Geometry check sheet. Reference: the model listing, model coordinates, mm. Face numbers are marked on the shaded views. A direction names the side the tool comes from. Give positions to 0.01 mm unless a question says otherwise; leave off trailing zeros. Order: outer loops, then holes, each group sorted by start corner. A loop starts at its lowest first (then second) coordinate and runs counter-clockwise, first axis right, second up. Notation, with made-up numbers: M 13.25,-3 L 64.25,-3 A28 ccw 64.25,31 Z; hole C -2.5,79 d11. An arc over 180 degrees is marked long. Answer as a JSON object with one key per item and string values. Group by question number.
from build123d import *

# Parameters (mm, degrees)
CROQUIS1_W                   = 90
CROQUIS1_H                   = 50.8
SALIENTE_EXTRUIR1_DEPTH      = 6.35
TALADRO_DE_MARGEN_PARA_M61_D = 6.6
CROQUIS4_W                   = 38.1
CROQUIS4_H                   = 12.7
SALIENTE_EXTRUIR2_DEPTH      = 134.38


with BuildPart() as part:
    # Croquis1 → Saliente-Extruir1 (new, symmetric)
    with BuildSketch(Plane(origin=(0, 0, 0), x_dir=(1, 0, 0), z_dir=(0, 1, 0))):
        Rectangle(CROQUIS1_W, CROQUIS1_H)
    extrude(amount=SALIENTE_EXTRUIR1_DEPTH, both=True)

    # Taladro de margen para M61 (through all)
    with Locations(Plane(origin=(0, -6.35, 0), x_dir=(-1, 0, 0), z_dir=(0, -1, 0))):
        with Locations((-36.583684882, -75.725395139), (-37, -17), (-37, 17), (-3, -17), (-3, 17)):
            Hole(TALADRO_DE_MARGEN_PARA_M61_D / 2)

    # Croquis4 → Saliente-Extruir2 (add)
    with BuildSketch(Plane(origin=(0, 6.35, 0), x_dir=(1, 0, 0), z_dir=(0, 1, 0))):
        with Locations((-25.95, 19.05)):
            Rectangle(CROQUIS4_W, CROQUIS4_H)
    extrude(amount=SALIENTE_EXTRUIR2_DEPTH)


solid = part.part
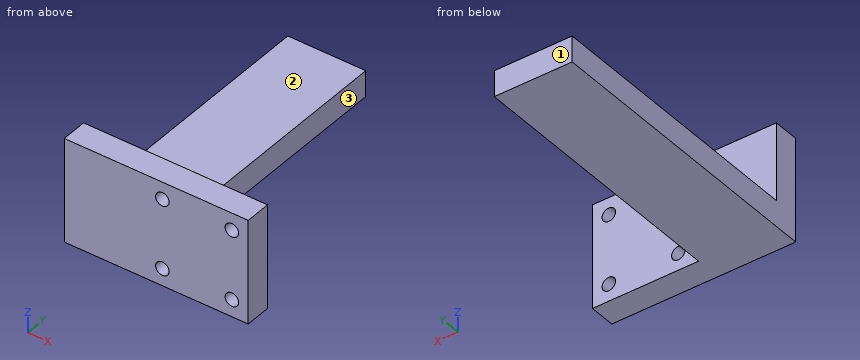
1. Thickness scan on line 1 along X through (y, z) = (2.5, 17); line 2 along Z through (x, y) = (37, 0); line 3 along X through (y, z) = (134, -17). Record the ranges inside material, lowest first. Write a range as [from, to].
2. Cross-section at A-A (z = -17). Record the cut outline in (x, y), and give its area (3 significant figures).
3. Access from +Z, -Z, +X, -X, +Y, -Y to the whole of each face (thin tool, end or side, straight path). Record for the marked faces 1, 2 and 3.
4. Cross-section at C-C (x = -18). Record the cut outline in (y, z), and give its area (3 significant figures).
5. Depth check by flat-ended pin: pin 1 (4 mm diameter, centred on x = 3, z = -17, fed in from +Y); pin 2 (10 mm diameter, centred on y = 43.5, z = -19.5, fed in from +X); pin 3 (7.5 mm diameter, centred on x = 37, z = -17, fed in from +Y); pin 4 (11.5 mm diameter, centred on x = -16.5, y = 98.5, fed in from +Z). Enter the tip coordinate at first touch or a pass-through.
6. Cross-section at B-B (x = 37). Record the cut outline in (y, z), and give its area (3 significant figures).
7. Cross-section at D-D (z = 17). Record the cut outline in (x, y).
Report:
{
 "1": {"line 1": "x = [-45, -0.3], [6.3, 33.7], [40.3, 45]", "line 2": "z = [-25.4, -20.3], [-13.7, 13.7], [20.3, 25.4]", "line 3": "x = [-45, -6.9]"},
 "2": {"outline": "M -45,-6.35 L -0.3,-6.35 L -0.3,6.35 L -6.9,6.35 L -6.9,140.73 L -45,140.73 Z; M 6.3,-6.35 L 33.7,-6.35 L 33.7,6.35 L 6.3,6.35 Z; M 40.3,-6.35 L 45,-6.35 L 45,6.35 L 40.3,6.35 Z", "area": "6,100 mm2"},
 "3": {"face 1": "+Z, -Z, +X, -X, +Y", "face 2": "+Z, +X, -X, +Y", "face 3": "+Z, -Z, +X, +Y"},
 "4": {"outline": "M -6.35,-25.4 L 140.73,-25.4 L 140.73,-12.7 L 6.35,-12.7 L 6.35,25.4 L -6.35,25.4 Z", "area": "2,350 mm2"},
 "5": {"pin 1": "passes through", "pin 2": "stops at x = -6.9", "pin 3": "stops at y = 6.35", "pin 4": "stops at z = -12.7"},
 "6": {"outline": "M -6.35,-25.4 L 6.35,-25.4 L 6.35,-20.3 L -6.35,-20.3 Z; M -6.35,-13.7 L 6.35,-13.7 L 6.35,13.7 L -6.35,13.7 Z; M -6.35,20.3 L 6.35,20.3 L 6.35,25.4 L -6.35,25.4 Z", "area": "478 mm2"},
 "7": {"outline": "M -45,-6.35 L -0.3,-6.35 L -0.3,6.35 L -45,6.35 Z; M 6.3,-6.35 L 33.7,-6.35 L 33.7,6.35 L 6.3,6.35 Z; M 40.3,-6.35 L 45,-6.35 L 45,6.35 L 40.3,6.35 Z"}
}
